Build history of the part. All positions in model axes, mm. A direction names the side the tool comes from. Round coordinates to 2 decimals unless told otherwise and drop trailing zeros. Order: outer loops, then holes, each group sorted by start corner. A loop starts at its lowest first (then second) coordinate and runs counter-clockwise, first axis right, second up. Notation, with made-up numbers: (1.5, 72.5) -> (31.5, 72.5) arc R16 cw to (31.5, 85.5) -> close; hole circle Ø6 at (32, 18.25). An arc over 180 degrees is marked (long way). Use a Markdown table: item, result. Add a question column.
Item 1: Two-plate mould, pull along Z, no slides. Class faces 1 (the face through (-4.48, -7.888, -244.798)), 2 (the face through (76, -16, -5)), 3 (the face through (-202, -8, 77.5)): released by +Z, released by -Z, zero draft, split by the parting line, or undercut.
Item 2: Slice it at B-B, the plane x = -120. Give the cut face in (y, z).
Item 3: 3-axis set-ups, long thin cutter, end or side, ignore diameter. For faces 4 (the face through (76, 0, -5)), 5 (the face through (-37.11, -8.11, -59.46)): which of +Z, -Z, +X, -X, +Y, -Y reach the whole face in a straight line?
Item 4: Slice it at C-C, the plane z = -223.5. Give the cut face in (x, y).
Item 5: Probe L1, parallel to X at y = -11, z = 127; L2, parallel to Z at x = 217, y = -7.5; L3, parallel to Z at x = 227.5, y = -4.75. List the from-to ranges inside material, lowest first.
Item 6: Slice it at D-D, the plane y = -10.5. State how many separate pieces and enclosed holes the cut face has, plus the area to 3 significant figures.
Item 7: Pin check, flat tips, straight feed: pin 1 (2 mm diameter, centred on x = -111, y = -5.5, fed in from -Z); pin 2 (6 mm diameter, centred on y = -8.5, z = 22.5, fed in from -X); pin 3 (4 mm diameter, centred on x = -43.5, y = -12.5, fed in from -Z). Stop position of each tip, or through.
Item 8: Slice it at A-A, the plane x = -48. Give the cut face in (y, z), plus the area to 3 significant figures.
from build123d import *

# Parameters (mm, degrees)
BOSS_EXTRUDE1_DEPTH = 16
FILLET1_R           = 60
SKETCH3_R           = 3.5
SKETCH3_R_2         = 4.25
SKETCH3_R_3         = 4.75
CUT_EXTRUDE1_DEPTH  = 475.506058971


with BuildPart() as part:
    # Sketch2 → Boss-Extrude1 (new body)
    with BuildSketch(Plane(origin=(0, 0, 0), x_dir=(1, 0, 0), z_dir=(0, 1, 0))):
        Polygon((-320, 142.5), (320, 350), (320, -350), (-320, -142.5), (-320, -77.5), (-20, -77.5), (-20, 77.5), (-320, 77.5), align=None)
    extrude(amount=-BOSS_EXTRUDE1_DEPTH)

    # Fillet1
    fillet1_edges = [part.edges().sort_by_distance(p)[0] for p in [
        (-20, -8, 77.5),
        (-20, -8, -77.5),
    ]]
    fillet(fillet1_edges, radius=FILLET1_R)

    # Sketch3 → Cut-Extrude1 (cut, through all)
    with BuildSketch(Plane(origin=(0, 0, 0), x_dir=(1, 0, 0), z_dir=(0, 1, 0))):
        with Locations(Location((45.573061117, 3.35862906, 0), (0, 0, 90))):
            Circle(SKETCH3_R)
        with Locations(Location((-231.09322879, -103.556104562, 0), (0, 0, 90))):
            Circle(SKETCH3_R_2)
        with Locations(Location((-298.17988721, -103.306000096, 0), (0, 0, 90))):
            Circle(SKETCH3_R_2)
        with Locations(Location((42.566176502, -157.759098005, 0), (0, 0, 90))):
            Circle(SKETCH3_R)
        with Locations(Location((36.930918819, -184.234632929, 0), (0, 0, 90))):
            Circle(SKETCH3_R)
        with Locations(Location((271.893921884, -229.22367877, 0), (0, 0, 90))):
            Circle(SKETCH3_R)
        with Locations(Location((189.782320405, -224.480960591, 0), (0, 0, 90))):
            Circle(SKETCH3_R)
        with Locations(Location((161.703177467, -193.571367621, 0), (0, 0, 90))):
            Circle(SKETCH3_R)
        with Locations(Location((165.959633732, -160.391798843, 0), (0, 0, 90))):
            Circle(SKETCH3_R)
        with Locations(Location((218.334544159, -129.392881806, 0), (0, 0, 90))):
            Circle(SKETCH3_R)
        with Locations(Location((284.479489307, -128.626354194, 0), (0, 0, 90))):
            Circle(SKETCH3_R)
        with Locations(Location((167.618318747, -46.69664923, 0), (0, 0, 90))):
            Circle(SKETCH3_R)
        with Locations(Location((162.099631238, -77.233713281, 0), (0, 0, 90))):
            Circle(SKETCH3_R)
        with Locations(Location((36.088570732, -73.915788734, 0), (0, 0, 90))):
            Circle(SKETCH3_R)
        with Locations(Location((42.875486949, -45.054299224, 0), (0, 0, 90))):
            Circle(SKETCH3_R)
        with Locations(Location((46.585239341, -9.907029228, 0), (0, 0, 90))):
            Circle(SKETCH3_R)
        with Locations(Location((-5.911515538, -10.255507999, 0), (0, 0, 90))):
            Circle(SKETCH3_R)
        with Locations(Location((65.684970424, 245.110909603, 0), (0, 0, 90))):
            Circle(SKETCH3_R_3)
        with Locations(Location((209.819274537, 289.932963664, 0), (0, 0, 90))):
            Circle(SKETCH3_R_3)
        with Locations(Location((-239.124203173, 102.548612385, 0), (0, 0, 90))):
            Circle(SKETCH3_R_2)
        with Locations(Location((-308.888078303, 102.548612385, 0), (0, 0, 90))):
            Circle(SKETCH3_R_2)
        with Locations(Location((42.566176502, 125.814947371, 0), (0, 0, 90))):
            Circle(SKETCH3_R)
        with Locations(Location((-11.908905398, 122.350563935, 0), (0, 0, 90))):
            Circle(SKETCH3_R)
        with Locations(Location((48.286557876, 110.984487849, 0), (0, 0, 90))):
            Circle(SKETCH3_R)
        with Locations(Location((-6.149033448, 109.550848491, 0), (0, 0, 90))):
            Circle(SKETCH3_R)
        with Locations(Location((-6.697602275, 5.835495982, 0), (0, 0, 90))):
            Circle(SKETCH3_R)
    extrude(amount=-CUT_EXTRUDE1_DEPTH, mode=Mode.SUBTRACT)


solid = part.part
Check sheet entries:
| question | item | result |
|---|---|---|
| 1 | face 1 | released by -Z |
| 1 | face 2 | zero draft |
| 1 | face 3 | undercut |
| 2 | outline | (-16, -207.34) -> (0, -207.34) -> (0, -77.5) -> (-16, -77.5) -> close; (-16, 77.5) -> (0, 77.5) -> (0, 207.34) -> (-16, 207.34) -> close |
| 3 | face 4 | +Z, -Z, +X, -X, +Y |
| 3 | face 5 | -X, +Y, -Y |
| 4 | outline | (-70.17, -16) -> (320, -16) -> (320, 0) -> (-70.17, 0) -> close |
| 5 | L1 | -320 to 215.78, 220.89 to 281.38, 287.58 to 320 |
| 5 | L2 | -316.61 to 126.16, 132.63 to 316.61 |
| 5 | L3 | -320.01 to 320.01 |
| 6 | separate pieces | 1 |
| 6 | enclosed holes | 26 |
| 6 | area | 269,000 mm2 |
| 7 | pin 1 | z = -210.59 |
| 7 | pin 2 | x = -20.54 |
| 7 | pin 3 | z = -232.79 |
| 8 | outline | (-16, -230.69) -> (0, -230.69) -> (0, -68.25) -> (-16, -68.25) -> close; (-16, 68.25) -> (0, 68.25) -> (0, 230.69) -> (-16, 230.69) -> close |
| 8 | area | 5,200 mm2 |
